Part model, mm, in its own coordinate system. A direction names the side the tool comes from. Round coordinates to 2 decimals unless told otherwise and drop trailing zeros. Write each loop counter-clockwise with the first axis right and the second up, starting at its lowest first coordinate (ties: lowest second). Pieces come first, ordered by that corner, then holes.
Autodesk Fusion 360 part; units mm, degrees
sketch "Sketch1" plane through (0, 0, 0) normal (0, 0, 1) x (1, 0, 0)
  line L0 (0, 0) -> (50, 0)
  line L1 (50, 0) -> (50, 25)
  line L2 (50, 25) -> (0, 25)
  line L3 (0, 25) -> (0, 0)
  line L4 (-2.5, -2.5) -> (52.5, -2.5)
  line L5 (52.5, -2.5) -> (52.5, 27.5)
  line L6 (52.5, 27.5) -> (-2.5, 27.5)
  line L7 (-2.5, 27.5) -> (-2.5, -2.5)
  line L8 (0, 25) -> (12.5, 25)
  line L9 (12.5, 25) -> (12.5, 12.5)
  line L10 (12.5, 12.5) -> (0, 12.5)
  line L11 (0, 12.5) -> (0, 25)
  line L12 (12.5, 12.5) -> (0, 12.5)
  line L13 (0, 12.5) -> (0, 0)
  line L14 (0, 0) -> (12.5, 0)
  line L15 (12.5, 0) -> (12.5, 12.5)
  line L16 (12.5, 12.5) -> (25, 12.5)
  line L17 (25, 12.5) -> (25, 25)
  line L18 (25, 25) -> (12.5, 25)
  line L19 (12.5, 25) -> (12.5, 12.5)
  line L20 (12.5, 12.5) -> (25, 12.5)
  line L21 (25, 12.5) -> (25, 0)
  line L22 (25, 0) -> (12.5, 0)
  line L23 (12.5, 0) -> (12.5, 12.5)
  line L24 (25, 12.5) -> (37.5, 12.5)
  line L25 (37.5, 12.5) -> (37.5, 25)
  line L26 (37.5, 25) -> (25, 25)
  line L27 (25, 25) -> (25, 12.5)
  line L28 (37.5, 12.5) -> (25, 12.5)
  line L29 (25, 12.5) -> (25, 0)
  line L30 (25, 0) -> (37.5, 0)
  line L31 (37.5, 0) -> (37.5, 12.5)
  line L32 (37.5, 12.5) -> (50, 12.5)
  line L33 (50, 12.5) -> (50, 0)
  line L34 (50, 0) -> (37.5, 0)
  line L35 (37.5, 0) -> (37.5, 12.5)
  line L36 (0, 25) -> (1, 25)
  line L37 (1, 25) -> (1, 0)
  line L38 (1, 0) -> (0, 0)
  line L39 (0, 0) -> (0, 25)
  line L40 (0, 25) -> (50, 25)
  line L41 (50, 25) -> (50, 24)
  line L42 (50, 24) -> (0, 24)
  line L43 (0, 24) -> (0, 25)
  line L44 (50, 0) -> (0, 0)
  line L45 (0, 0) -> (0, 1)
  line L46 (0, 1) -> (50, 1)
  line L47 (50, 1) -> (50, 0)
  line L48 (50, 25) -> (49, 25)
  line L49 (49, 25) -> (49, 0)
  line L50 (49, 0) -> (50, 0)
  line L51 (50, 0) -> (50, 25)
  line L52 (0, 12.5) -> (50, 12.5)
  line L53 (50, 12.5) -> (50, 11.5)
  line L54 (50, 11.5) -> (0, 11.5)
  line L55 (0, 11.5) -> (0, 12.5)
  line L56 (0, 12.5) -> (50, 12.5)
  line L57 (50, 12.5) -> (50, 13.5)
  line L58 (50, 13.5) -> (0, 13.5)
  line L59 (0, 13.5) -> (0, 12.5)
  line L60 (50, 25) -> (49, 25)
  line L61 (49, 25) -> (49, 0)
  line L62 (49, 0) -> (50, 0)
  line L63 (50, 0) -> (50, 25)
  line L64 (12.5, 0) -> (13.5, 0)
  line L65 (13.5, 0) -> (13.5, 25)
  line L66 (13.5, 25) -> (12.5, 25)
  line L67 (12.5, 25) -> (12.5, 0)
  line L68 (12.5, 25) -> (11.5, 25)
  line L69 (11.5, 25) -> (11.5, 0)
  line L70 (11.5, 0) -> (12.5, 0)
  line L71 (12.5, 0) -> (12.5, 25)
  line L72 (25, 25) -> (26, 25)
  line L73 (26, 25) -> (26, 0)
  line L74 (26, 0) -> (25, 0)
  line L75 (25, 0) -> (25, 25)
  line L76 (25, 25) -> (24, 25)
  line L77 (24, 25) -> (24, 0)
  line L78 (24, 0) -> (25, 0)
  line L79 (25, 0) -> (25, 25)
  line L80 (37.5, 25) -> (38.5, 25)
  line L81 (38.5, 25) -> (38.5, 0)
  line L82 (38.5, 0) -> (37.5, 0)
  line L83 (37.5, 0) -> (37.5, 25)
  line L84 (37.5, 25) -> (36.5, 25)
  line L85 (36.5, 25) -> (36.5, 0)
  line L86 (36.5, 0) -> (37.5, 0)
  line L87 (37.5, 0) -> (37.5, 25)
  line L88 (1, 24) -> (11.5, 13.5)
  line L89 (1, 13.5) -> (11.5, 24)
  line L90 (1, 11.5) -> (11.5, 1)
  line L91 (1, 1) -> (11.5, 11.5)
  line L92 (13.5, 24) -> (24, 13.5)
  line L93 (13.5, 13.5) -> (24, 24)
  line L94 (13.5, 11.5) -> (24, 1)
  line L95 (13.5, 1) -> (24, 11.5)
  line L96 (26, 11.5) -> (36.5, 1)
  line L97 (26, 1) -> (26, 1.4048)
  line L98 (36.5, 11.5) -> (26, 1)
  line L99 (36.5, 24) -> (26, 13.5)
  line L100 (26, 24) -> (36.5, 13.5)
  line L101 (38.5, 24) -> (49, 13.5)
  line L102 (38.5, 13.5) -> (49, 24)
  line L103 (38.5, 11.5) -> (49, 1)
  line L104 (38.5, 1) -> (49, 11.5)
  circle A0 centre (6.25, 18.75) radius 2.5
  circle A1 centre (18.75, 18.75) radius 2.5
  circle A2 centre (31.25, 18.75) radius 2.5
  circle A3 centre (43.75, 18.75) radius 2.5
  circle A4 centre (43.75, 6.25) radius 2.5
  circle A5 centre (31.25, 6.25) radius 2.5
  circle A6 centre (18.75, 6.25) radius 2.5
  circle A7 centre (6.25, 6.25) radius 2.5
  circle A8 centre (18.75, 6.25) radius 3.5
  circle A9 centre (31.25, 6.25) radius 3.5
  circle A10 centre (31.25, 18.75) radius 3.5
  circle A11 centre (18.75, 18.75) radius 3.5
  circle A12 centre (6.25, 18.75) radius 3.5
  circle A13 centre (43.75, 18.75) radius 3.5
  circle A14 centre (6.25, 6.25) radius 3.5
  circle A15 centre (43.75, 6.25) radius 3.5
  dimension "d1" = 50
  dimension "d2" = 25
  dimension "d3" = 2.5
  dimension "d4" = 12.5
  dimension "d5" = 12.5
  dimension "d6" = 12.5
  dimension "d7" = 12.5
  dimension "d8" = 12.5
  dimension "d9" = 12.5
  dimension "d10" = 12.5
  dimension "d11" = 12.5
  dimension "d12" = 12.5
  dimension "d13" = 12.5
  dimension "d14" = 12.5
  dimension "d15" = 1
  dimension "d16" = 1
  dimension "d17" = 1
  dimension "d18" = 1
  dimension "d19" = 25
  dimension "d20" = 50
  dimension "d21" = 1
  dimension "d22" = 50
  dimension "d23" = 1
  dimension "d24" = 1
  dimension "d25" = 1
  dimension "d26" = 25
  dimension "d27" = 1
  dimension "d28" = 1
  dimension "d29" = 1
  dimension "d30" = 1
  dimension "d31" = 5
  dimension "d32" = 5
  dimension "d33" = 5
  dimension "d34" = 5
  dimension "d35" = 5
  dimension "d36" = 5
  dimension "d37" = 5
  dimension "d38" = 5
  dimension "d39" = 1
  dimension "d40" = 1
  dimension "d41" = 1
  dimension "d42" = 1
  dimension "d43" = 1
  dimension "d44" = 1
  dimension "d51" = 1
  dimension "d52" = 1
extrude "Extrude2" add sketch "Sketch1" along normal blind 5 contours L0 L3 L13 L14 L37 L38 L39 L44 L45 L46 | L0 L14 L37 L44 L46 L69 | L3 L13 L37 L39 L46 L54 | L0 L14 L15 L23 L44 L46 L67 L69 L70 L71 | L3 L10 L12 L13 L37 L39 L52 L54 L55 L56 | L0 L15 L22 L23 L44 L46 L64 L65 L67 L71 | L15 L23 L46 L54 L67 L69 L71 | L10 L12 L37 L52 L54 L56 L69 | L3 L10 L11 L12 L37 L39 L52 L56 L58 L59 | L0 L22 L44 L46 L65 L77 | L15 L23 L46 L54 L65 L67 L71 | L10 L12 L15 L23 L52 L54 L56 L67 L69 L71 | L10 L12 L37 L52 L56 L58 L69 | L3 L11 L37 L39 L42 L58 | L0 L21 L22 L29 L44 L46 L75 L77 L78 L79 | L15 L16 L20 L23 L52 L54 L56 L65 L67 L71 | L9 L10 L12 L19 L52 L56 L58 L67 L69 L71 | L2 L3 L8 L11 L36 L37 L39 L40 L42 L43 | L0 L21 L29 L30 L44 L46 L73 L74 L75 L79 | L21 L29 L46 L54 L75 L77 L79 | L16 L20 L52 L54 L56 L65 L77 | L9 L16 L19 L20 L52 L56 L58 L65 L67 L71 | L9 L19 L42 L58 L67 L69 L71 | L2 L8 L37 L40 L42 L69 | L0 L30 L44 L46 L73 L85 | L21 L29 L46 L54 L73 L75 L79 L97 | L16 L20 L21 L29 L52 L54 L56 L75 L77 L79 | L16 L20 L52 L56 L58 L65 L77 | L9 L19 L42 L58 L65 L67 L71 | L2 L8 L9 L19 L40 L42 L67 L68 L69 L71 | L0 L30 L31 L35 L44 L46 L83 L85 L86 L87 | L21 L24 L28 L29 L52 L54 L56 L73 L75 L79 | L16 L17 L20 L27 L52 L56 L58 L75 L77 L79 | L2 L9 L18 L19 L40 L42 L65 L66 L67 L71 | L0 L31 L34 L35 L44 L46 L81 L82 L83 L87 | L31 L35 L46 L54 L83 L85 L87 | L17 L24 L27 L28 L52 L56 L58 L73 L75 L79 | L24 L28 L52 L54 L56 L73 L85 | L17 L27 L42 L58 L75 L77 L79 | L2 L18 L40 L42 L65 L77 | L0 L34 L44 L46 L49 L61 L81 | L31 L35 L46 L54 L81 L83 L87 | L24 L28 L31 L35 L52 L54 L56 L83 L85 L87 | L17 L27 L42 L58 L73 L75 L79 | L24 L28 L52 L56 L58 L73 L85 | L2 L17 L18 L27 L40 L42 L75 L76 L77 L79 | L0 L1 L33 L34 L44 L46 L47 L49 L50 L51 L61 L62 L63 | L31 L32 L35 L52 L54 L56 L81 L83 L87 | L24 L25 L28 L52 L56 L58 L83 L85 L87 | L2 L17 L26 L27 L40 L42 L72 L73 L75 L79 | L1 L33 L46 L49 L51 L54 L61 L63 | L32 L49 L52 L54 L56 L61 L81 | L25 L32 L52 L56 L58 L81 L83 L87 | L25 L42 L58 L83 L85 L87 | L2 L26 L40 L42 L73 L85 | L1 L32 L33 L49 L51 L52 L53 L54 L56 L61 L63 | L32 L49 L52 L56 L58 L61 L81 | L25 L42 L58 L81 L83 L87 | L2 L25 L26 L40 L42 L83 L84 L85 L87 | L1 L32 L49 L51 L52 L56 L57 L58 L61 L63 | L2 L25 L40 L42 L80 L81 L83 L87 | L1 L42 L49 L51 L58 L61 L63 | L2 L40 L42 L49 L61 L81 | L1 L2 L40 L41 L42 L48 L49 L51 L60 L61 L63 makes body 1
extrude "Extrude1" add sketch "Sketch1" along normal blind 2 separate body contours L90 L91 A7 A14 | L90 L91 A7 A14 | L90 L91 A7 A14 | L90 L91 A7 A14 | L94 L95 A6 A8 | L94 L95 A6 A8 | L88 L89 A0 A12 | L88 L89 A0 A12 | L94 L95 A6 A8 | L94 L95 A6 A8 | L88 L89 A0 A12 | L88 L89 A0 A12 | L96 L98 A5 A9 | L96 L98 A5 A9 | L92 L93 A1 A11 | L92 L93 A1 A11 | L96 L98 A5 A9 | L96 L98 A5 A9 | L92 L93 A1 A11 | L92 L93 A1 A11 | L103 L104 A4 A15 | L103 L104 A4 A15 | L99 L100 A2 A10 | L99 L100 A2 A10 | L103 L104 A4 A15 | L103 L104 A4 A15 | L99 L100 A2 A10 | L99 L100 A2 A10 | L101 L102 A3 A13 | L101 L102 A3 A13 | L101 L102 A3 A13 | L101 L102 A3 A13 makes body 2 at (9.7326, 19.0985, 1.3333) makes body 3 at (34.7326, 6.5985, 0.6667) makes body 4 at (22.2326, 19.0985, 1.3333) makes body 5 at (34.7326, 19.0985, 0.6667) makes body 6 at (22.2326, 6.5985, 0.6667) makes body 7 at (47.2326, 6.5985, 1.3333) makes body 8 at (47.2326, 19.0985, 1.3333) makes body 9 at (9.7326, 6.5985, 1.3333)
extrude "Extrude3" add sketch "Sketch1" along normal blind 1 contours L37 L90 L91 A14 | L69 L90 L91 A14 | L90 L91 A7 A14 | L90 L91 A7 A14 | L65 L94 L95 A8 | L37 L88 L89 A12 | L77 L94 L95 A8 | L69 L88 L89 A12 | L73 L96 L97 L98 A9 | L65 L92 L93 A11 | L85 L96 L98 A9 | L77 L92 L93 A11 | L81 L103 L104 A15 | L73 L99 L100 A10 | L49 L61 L103 L104 A15 | L103 L104 A4 A15 | L85 L99 L100 A10 | L103 L104 A4 A15 | L81 L101 L102 A13 | L49 L61 L101 L102 A13 picked at (3.824, 4.2265) picked at (9.3996, 5.9889) picked at (41.0607, 4.5923) picked at (46.0898, 4.1256) bodies 7 1 3 4 5 6 8 9 2
Q1. Drop flat-ended pins along their axis: P1, Ø8, axis at x = 20.5, y = 6, coming from the +Z side; P2, Ø1.4, axis at x = 10, y = 18.5, coming from the +Z side; P3, Ø0.8, axis at x = 27, y = 9, coming from the +Z side; P4, Ø3, axis at x = 6.25, y = 18.75, coming from the -Z side. Give the stop position or say it passes through.
Q2. Wall check: line 1 (Y direction, x = 8, z = 3.6); line 2 (X direction, y = 8.25, z = 2.7); line 3 (Z direction, x = 35.5, y = 14.75). Give the ranges that are in metal, low to high.
Q3. Saw through at B-B, the plane y = 18.75. Give the number of separate pieces and of enclosed holes in the cut face, and give its area (3 significant figures).
Q4. Saw through at A-A, the plane x = 31.25. Write the cut outline in (y, z).
Q5. Tool access for faces 1 (the flat face through (23, 13, 5)), 2 (the flat face through (40, 6, 1)), 3 (the flat face through (6, 11.5, 2)): list every direction of +Z, -Z, +X, -X, +Y, -Y with a clear straight run to the whole face (end or side of a thin tool).
Q6. Saw through at D-D, the plane x = 18. Write the cut outline in (y, z).
Computed:
1. P1: stops at z = 5
1. P2: stops at z = 2
1. P3: stops at z = 1
1. P4: passes through
2. line 1: y = 0 to 1, 11.5 to 13.5, 24 to 25
2. line 2: x = 0 to 1, 11.5 to 13.5, 24 to 26, 36.5 to 38.5, 49 to 50
2. line 3: z = 0 to 1
3. separate pieces: 5
3. enclosed holes: 0
3. area: 70.0 mm2
4. outline: (0, 0) - (1, 0) - (1, 5) - (0, 5) - close; (2.75, 0) - (3.75, 0) - (3.75, 2) - (2.75, 2) - close; (8.75, 0) - (9.75, 0) - (9.75, 2) - (8.75, 2) - close; (11.5, 0) - (13.5, 0) - (13.5, 5) - (11.5, 5) - close; (15.25, 0) - (16.25, 0) - (16.25, 2) - (15.25, 2) - close; (21.25, 0) - (22.25, 0) - (22.25, 2) - (21.25, 2) - close; (24, 0) - (25, 0) - (25, 5) - (24, 5) - close
5. face 1: +Z, +X, -X, +Y, -Y
5. face 2: +Z
5. face 3: +Z, -Z
6. outline: (0, 0) - (1, 0) - (1, 5) - (0, 5) - close; (2.83, 0) - (3.87, 0) - (3.87, 2) - (2.83, 2) - close; (8.63, 0) - (9.67, 0) - (9.67, 2) - (8.63, 2) - close; (11.5, 0) - (13.5, 0) - (13.5, 5) - (11.5, 5) - close; (15.33, 0) - (16.37, 0) - (16.37, 2) - (15.33, 2) - close; (21.13, 0) - (22.17, 0) - (22.17, 2) - (21.13, 2) - close; (24, 0) - (25, 0) - (25, 5) - (24, 5) - close
